```python
from build123d import *

# Parameters (mm, degrees)
SKETCH1_R           = 14
BOSS_EXTRUDE1_DEPTH = 19
SKETCH2_W           = 14.6
SKETCH2_H           = 5.495823158
BOSS_EXTRUDE2_DEPTH = 19
SKETCH3_R           = 2.1
BOSS_EXTRUDE3_DEPTH = 2
SKETCH4_R           = 2.5
BOSS_EXTRUDE4_DEPTH = 10


with BuildPart() as part:
    # Sketch1 → Boss-Extrude1 (new body)
    with BuildSketch(Plane(origin=(0, 0, 0), x_dir=(1, 0, 0), z_dir=(0, 1, 0))):
        with Locations(Location((0, 0, 0), (0, 0, 270))):
            Circle(SKETCH1_R)
    extrude(amount=BOSS_EXTRUDE1_DEPTH)

    # Sketch2 → Boss-Extrude2 (add)
    with BuildSketch(Plane(origin=(0, 19, 0), x_dir=(1, 0, 0), z_dir=(0, 1, 0))):
        with Locations((0, -14.252088421)):
            Rectangle(SKETCH2_W, SKETCH2_H)
    extrude(amount=-BOSS_EXTRUDE2_DEPTH)

    # Sketch3 → Boss-Extrude3 (add)
    # profile 1 of 2: a face of its own
    with BuildSketch(Plane(origin=(0, 19, 0), x_dir=(1, 0, 0), z_dir=(0, 1, 0))):
        with BuildLine():
            Line((-17.5, 3.5), (-12.399863738, 3.5))
            Line((-12.399863738, 3.5), (-12.399863738, -3.5))
            Line((-12.399863738, -3.5), (-17.5, -3.5))
            ThreePointArc((-17.5, -3.5), (-21, 0), (-17.5, 3.5))
        make_face()
        with Locations(Location((-17.5, 0, 0), (0, 0, 270))):
            Circle(SKETCH3_R, mode=Mode.SUBTRACT)
    # profile 2 of 2: a face of its own
    with BuildSketch(Plane(origin=(0, 19, 0), x_dir=(1, 0, 0), z_dir=(0, 1, 0))):
        with BuildLine():
            Line((12.399863738, -3.5), (17.5, -3.5))
            ThreePointArc((17.5, -3.5), (21, 0), (17.5, 3.5))
            Line((17.5, 3.5), (12.399863738, 3.5))
            Line((12.399863738, 3.5), (12.399863738, -3.5))
        make_face()
        with Locations(Location((17.5, 0, 0), (0, 0, 90))):
            Circle(SKETCH3_R, mode=Mode.SUBTRACT)
    extrude(amount=-BOSS_EXTRUDE3_DEPTH)

    # Sketch4 → Boss-Extrude4 (add)
    with BuildSketch(Plane(origin=(0, 19, 0), x_dir=(1, 0, 0), z_dir=(0, 1, 0))):
        with Locations(Location((0, 8, 0), (0, 0, 270))):
            Circle(SKETCH4_R)
    extrude(amount=BOSS_EXTRUDE4_DEPTH)


solid = part.part
```
Geometry: final body of the model. Coordinates: model frame, mm. A direction names the side the tool comes from. Coordinates: 2 decimals unless noted, no trailing zeros. Order: outer loops, then holes, each group sorted by start corner. A loop starts at its lowest first (then second) coordinate and runs counter-clockwise, first axis right, second up. Notation, with made-up numbers: (-11.75, 11.5) - (21.25, 11.5) arc R20 cw to (21.25, 28.5) - close; hole circle Ø7 at (9, 60). An arc over 180 degrees is marked (long way). Return JSON: item names as keys, results as strings. Group by question number.
1. Cut plane D-D (y = 9). Output: boundary loops of the cut face in (x, z).
2. Set-up query: faces 1 (the face through (16, 18, -3.5)), 2 (the face through (7.3, 10, 15)), 3 (the face through (-7.3, 10, 15)), 4 (the face through (-16, 18, -3.5)). Return all of +Z, -Z, +X, -X, +Y, -Y with unobstructed straight access to the full face (end or side cutting, diameter ignored); none if empty.
3. Material intervals for line 1 along X through (y, z) = (18.45, 0); line 2 along Z through (x, y) = (17.5, 17.7); line 3 along Y through (x, z) = (12, 4), sorted ascending. Write a range as [from, to].
4. Cut plane A-A (x = 0). Output: boundary loops of the cut face in (y, z).
5. Pin query (flat end, axial travel): pin 1 (2 mm diameter, centred on y = 25, z = -9.5, fed in from +X); pin 2 (5 mm diameter, centred on x = 17.5, z = 0, fed in from -Y); pin 3 (1 mm diameter, centred on x = 15.5, y = 18, fed in from -Z); pin 4 (1 mm diameter, centred on x = 7.5, z = 10, fed in from -Y). Return the tip coordinate at first contact, or that it passes through.
6. Cut plane B-B (z = -7.5). Output: boundary loops of the cut face in (x, y).
7. Cut plane C-C (y = 25). Output: boundary loops of the cut face in (x, z), plus the area to 3 significant figures.
Resolved:
{
 "1": {"outline": "(-7.3, 11.95) arc R14 ccw (long way) to (7.3, 11.95) - (7.3, 17) - (-7.3, 17) - close"},
 "2": {"face 1": "-Z, +X, +Y, -Y", "face 2": "+Z, +X, +Y, -Y", "face 3": "+Z, -X, +Y, -Y", "face 4": "-Z, -X, +Y, -Y"},
 "3": {"line 1": "x = [-21, -19.6], [-15.4, 15.4], [19.6, 21]", "line 2": "z = [-3.5, -2.1], [2.1, 3.5]", "line 3": "y = [0, 19]"},
 "4": {"outline": "(0, -14) - (19, -14) - (19, -10.5) - (29, -10.5) - (29, -5.5) - (19, -5.5) - (19, 17) - (0, 17) - close"},
 "5": {"pin 1": "stops at x = 2.45", "pin 2": "stops at y = 17", "pin 3": "stops at z = -3.5", "pin 4": "stops at y = 0"},
 "6": {"outline": "(-11.82, 0) - (11.82, 0) - (11.82, 19) - (2.45, 19) - (2.45, 29) - (-2.45, 29) - (-2.45, 19) - (-11.82, 19) - close"},
 "7": {"outline": "circle Ø5 at (0, -8)", "area": "19.6 mm²"}
}
